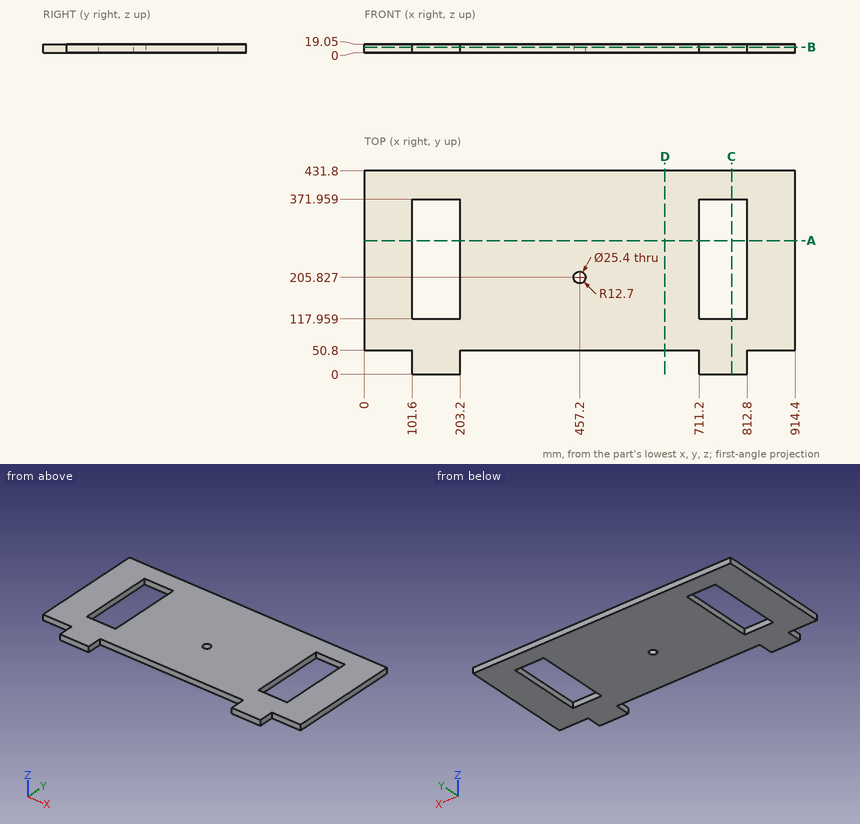
Here's the drawing with two shaded views (mm, measured from the low corner). I have some questions. Coordinates: 2 decimals unless noted, no trailing zeros. Loops run counter-clockwise (first coordinate to the right, second up) from the corner with the lowest first, then second, coordinate; pieces in that order, holes last. Notation, with made-up numbers: (-34, 74) -> (-28, 74) arc R26 cw to (-28, 100) -> close; hole circle Ø8 at (69.5, 65). An arc over 180 degrees is marked (long way). Put each result on its own line as item: value. Start each with the question number.
Q1. I want a section at D-D (x = 638). Write out the boundary of the cut face in (y, z).
Q2. If I drill on line 1 (X direction, y = 188, z = 7.5); line 2 (Y direction, x = 131.5, z = 7.25); line 3 (X direction, y = 44, z = 16.75), over which ranges is the centre line in solid material (lowest first)? Write a range as [from, to].
Q3. I want a section at C-C (x = 780). Write out the boundary of the cut face in (y, z).
Q4. I want a section at A-A (y = 284). Write out the boundary of the cut face in (x, z).
Q5. I want a section at B-B (z = 12.5). Write out the boundary of the cut face in (x, y), plus the area to 3 significant figures.
Q6. I'm going to push flat-ended pins straight in: P1, Ø9.5, axis at y = 305.5, z = 6.5, coming from the -X side; P2, Ø6, axis at y = 45.5, z = 14, coming from the -X side; P3, Ø15, axis at x = 457.2, y = 205.83, coming from the -Z side; P4, Ø9.5, axis at y = 19.5, z = 13.5, coming from the +X side. Where does each tip first touch, or does it pass through?
Taken from the geometry:
1. outline: (50.8, 0) -> (431.8, 0) -> (431.8, 19.05) -> (50.8, 19.05) -> close
2. line 1: x = [0, 101.6], [203.2, 711.2], [812.8, 914.4]
2. line 2: y = [0, 117.96], [371.96, 431.8]
2. line 3: x = [101.6, 203.2], [711.2, 812.8]
3. outline: (0, 0) -> (117.96, 0) -> (117.96, 19.05) -> (0, 19.05) -> close; (371.96, 0) -> (431.8, 0) -> (431.8, 19.05) -> (371.96, 19.05) -> close
4. outline: (0, 0) -> (101.6, 0) -> (101.6, 19.05) -> (0, 19.05) -> close; (203.2, 0) -> (711.2, 0) -> (711.2, 19.05) -> (203.2, 19.05) -> close; (812.8, 0) -> (914.4, 0) -> (914.4, 19.05) -> (812.8, 19.05) -> close
5. outline: (0, 50.8) -> (101.6, 50.8) -> (101.6, 0) -> (203.2, 0) -> (203.2, 50.8) -> (711.2, 50.8) -> (711.2, 0) -> (812.8, 0) -> (812.8, 50.8) -> (914.4, 50.8) -> (914.4, 431.8) -> (0, 431.8) -> close; hole (101.6, 117.96) -> (203.2, 117.96) -> (203.2, 371.96) -> (101.6, 371.96) -> close; hole circle Ø25.4 at (457.2, 205.83); hole (711.2, 117.96) -> (812.8, 117.96) -> (812.8, 371.96) -> (711.2, 371.96) -> close
5. area: 307,000 mm2
6. P1: stops at x = 0
6. P2: stops at x = 101.6
6. P3: passes through
6. P4: stops at x = 812.8
